Autodesk Fusion 360 part; units mm, degrees
sketch "Sketch1" plane through (0, 0, 0) normal (0, 1, 0) x (1, 0, 0)
  line L0 (-18.22, -14.04) -> (0, -14.04)
  line L1 (0, -14.04) -> (0, 14.04)
  line L2 (0, 14.04) -> (-18.22, 14.04)
  line L3 (-18.22, 14.04) -> (-18.22, -14.04)
  line L4 (0, -5.075) -> (-4, -5.075)
  line L5 (-4, -5.075) -> (-4, -7.75)
  line L6 (-4, -7.75) -> (-14.22, -7.75)
  line L7 (0, 5.075) -> (-4, 5.075)
  line L8 (-4, 5.075) -> (-4, 7.75)
  line L9 (-4, 7.75) -> (-14.22, 7.75)
  line L10 (-14.22, 7.75) -> (-14.22, -7.75)
  line L11 (-18.22, 0) -> (0, 0) construction
  line L12 (-4, -5.075) -> (-4, 5.075) construction
  point P0 (-14.22, 0)
  point P1 (-4, 0)
  dimension "d1" = 28.08
  dimension "d2" = 10.15
  dimension "d3" = 4
  dimension "d4" = 10.22
  dimension "d5" = 15.5
  dimension "d6" = 2.675
  dimension "d7" = 14.22
  dimension "d10" = 4
extrude "Extrude1" add sketch "Sketch1" along normal blind 100 contours L0 L1 L2 L3 L4 L5 L6 L7 L8 L9 L10 makes body 1
sketch "Sketch2" plane through (0, 0, 0) normal (0, 1, 0) x (1, 0, 0)
  line L0 (-4, -7.75) -> (-14.22, -7.75)
  line L1 (-14.22, 7.75) -> (-14.22, -7.75)
  line L2 (-4, 7.75) -> (-14.22, 7.75)
  line L3 (-4, 5.075) -> (-4, 7.75)
  line L4 (0, 5.075) -> (-4, 5.075)
  line L5 (0, -5.075) -> (-4, -5.075)
  line L6 (-4, -5.075) -> (-4, -7.75)
  line L7 (0, -14.04) -> (0, 14.04)
  line L8 (0, 5.075) -> (0, -5.075)
  line L9 (-0.4, -4.675) -> (-4.4, -4.675)
  line L10 (-4.4, -4.675) -> (-4.4, -7.35)
  line L11 (-4.4, -7.35) -> (-13.82, -7.35)
  line L12 (-13.82, 7.35) -> (-13.82, -7.35)
  line L13 (-4.4, 7.35) -> (-13.82, 7.35)
  line L14 (-4.4, 4.675) -> (-4.4, 7.35)
  line L15 (-0.4, 4.675) -> (-4.4, 4.675)
  line L16 (-0.4, 4.675) -> (-0.4, -4.675)
  dimension "d11" = 0.4
extrude "Extrude2" add sketch "Sketch2" along normal mid plane 20 separate body contours L9 L10 L11 L12 L13 L14 L15 L16 makes body 2
sketch "Sketch4" plane through (-13.82, 0, 0) normal (-1, 0, 0) x (0, -1, 0)
  line L0 (10, 7.35) -> (-10, 7.35)
  line L1 (-10, 7.35) -> (-10, -7.35)
  line L2 (-10, -7.35) -> (10, -7.35)
  line L3 (10, -7.35) -> (10, 7.35)
  line L4 (3.3811, 5.8563) -> (-3.3811, 5.8562)
  line L5 (-3.3811, 5.8562) -> (-6.7622, 0)
  line L6 (-6.7622, 0) -> (-3.3811, -5.8563)
  line L7 (-3.3811, -5.8563) -> (3.3811, -5.8563)
  line L8 (3.3811, -5.8563) -> (6.7622, 0)
  line L9 (6.7622, 0) -> (3.3811, 5.8563)
  line L10 (0, 0) -> (10, 0) construction
  circle A0 centre (0, 0) radius 3.378
  dimension "d14" = 11.7125
  dimension "d23" = 6.756
extrude "Extrude3" cut sketch "Sketch4" against normal blind 6.5563 contours L4 L5 L6 L7 L8 L9 bodies 2
extrude "Extrude4" cut sketch "Sketch4" against normal blind 25.66 contours A0 bodies 2
chamfer "Chamfer1" distance 0.4 angle 45 23 edges at (-9.11, 10, 7.35) (-4.4, 0, 7.35) (-9.11, -10, 7.35) (-4.4, 10, 6.0125) (-2.4, 10, 4.675) (-0.4, 10, 0) (-2.4, 10, -4.675) (-4.4, 10, -6.0125) (-9.11, 10, -7.35) (-4.4, 0, -7.35) (-4.4, -10, 6.0125) (-2.4, -10, 4.675) (-0.4, -10, 0) (-2.4, -10, -4.675) (-4.4, -10, -6.0125) (-9.11, -10, -7.35) (-0.4, 0, 4.675) (-0.4, 0, -4.675) (-0.4, 3.1494, -1.2215) (-13.82, 0, 7.35) (-13.82, -10, 0) (-13.82, 0, -7.35) (-13.82, 10, 0) on bodies 2
chamfer "Chamfer2" distance 0.4 angle 45 6 edges at (-13.82, 5.0717, 2.9281) (-13.82, 0, 5.8563) (-13.82, -5.0717, 2.9281) (-13.82, -5.0717, -2.9281) (-13.82, 0, -5.8563) (-13.82, 5.0717, -2.9281) on bodies 2
sketch "Sketch5" plane through (-7.2638, 0, 0) normal (-1, 0, 0) x (0, -1, 0)
  circle A0 centre (0, 0) radius 3.378
  line L0 (6.7622, 0) -> (3.3811, 5.8563)
  line L1 (3.3811, 5.8563) -> (-3.3811, 5.8562)
  line L2 (-3.3811, 5.8562) -> (-6.7622, 0)
  line L3 (-6.7622, 0) -> (-3.3811, -5.8563)
  line L4 (-3.3811, -5.8563) -> (3.3811, -5.8563)
  line L5 (3.3811, -5.8563) -> (6.7622, 0)
extrude "Extrude5" add sketch "Sketch5" against normal blind 0.2 contours A0 bodies 2
hidden bodies 1
equation "d14 = 7 in / 16 + 0.6 mm"
equation "d15 = -7 in / 32 - 1 mm"
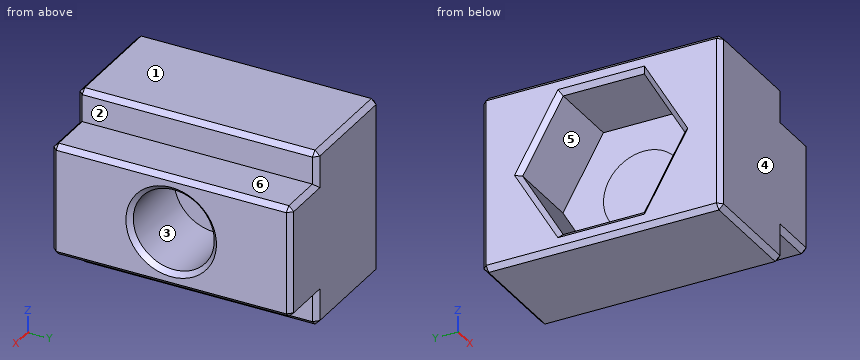
The listing builds one solid part. Answer for the finished solid, in the listing's coordinates (mm). Face numbers are marked on the shaded views. A direction names the side the tool comes from. Give positions to 0.01 mm unless a question says otherwise; leave off trailing zeros. Order: outer loops, then holes, each group sorted by start corner. A loop starts at its lowest first (then second) coordinate and runs counter-clockwise, first axis right, second up. Notation, with made-up numbers: (55, 78.5) - (97, 78.5) arc R24 cw to (97, 91.5) - close; hole circle Ø5 at (71, 50). An arc over 180 degrees is marked (long way). One line per item, written item: value. Start each with the question number.
1) Find the intervals of material crossed by L1, parallel to Z at x = -3.25, y = 0 (3 decimals); L2, parallel to Z at x = -8.25, y = 1; L3, parallel to X at y = -3, z = 3, in increasing order.
2) A cutting plane is placed at C-C on z = 5. Give the vertices of the cut face in (x, y).
3) A tool of negligible diameter and unlimited length cuts with its end or side. For the marked faces 1, 2 and 3, from which of +Z, -Z, +X, -X, +Y, -Y can it reach the whole face along a straight path? Write none if from no direction.
4) A cutting plane is placed at D-D on x = -6.5. Give the vertices of the cut face in (y, z), then the cut area to 3 significant figures.
5) Given pin 1 Ø1.8 at (x, y) = (-2, -2.5) entering from -Z (3 decimals); pin 2 Ø3.5 at (y, z) = (1, -1) entering from -X; pin 3 Ø0.7 at (y, z) = (1.5, -5.5) entering from +X, each flat-ended and moving along its own axis, determine where each tip first touches the part or whether it passes through.
6) A cutting plane is placed at A-A on x = -3. Give the vertices of the cut face in (y, z) (3 decimals).
7) The mould has two halves that part along Y. Classify the marked faces 4, 5 and 6: released by +Y, released by -Y, zero draft, split by the parting line, or undercut.
8) A cutting plane is placed at B-B on y = 0. Give the vertices of the cut face in (x, z) (3 decimals).
Answer sheet:
1. L1: z = -4.675 to -3.378, 3.378 to 4.675
1. L2: z = -7.35 to -5.86, 5.86 to 7.35
1. L3: x = -7.26 to -0.4
2. outline: (-13.82, -9.6) - (-13.42, -10) - (-4.8, -10) - (-4.4, -9.6) - (-4.4, 9.6) - (-4.8, 10) - (-13.42, 10) - (-13.82, 9.6) - (-13.82, 4.34) - (-13.42, 3.88) - (-7.26, 3.88) - (-7.26, -3.88) - (-13.42, -3.88) - (-13.82, -4.34) - close
3. face 1: +Z, +X, -X, +Y, -Y
3. face 2: +Z, +X, +Y, -Y
3. face 3: +X
4. outline: (-10, -6.95) - (-9.6, -7.35) - (9.6, -7.35) - (10, -6.95) - (10, 6.95) - (9.6, 7.35) - (-9.6, 7.35) - (-10, 6.95) - close; hole circle Ø6.76 at (0, 0)
4. area: 258 mm2
5. pin 1: stops at z = -4.675
5. pin 2: stops at x = -7.26
5. pin 3: stops at x = -4.4
6. outline: (-10, -4.275) - (-9.6, -4.675) - (9.6, -4.675) - (10, -4.275) - (10, 4.275) - (9.6, 4.675) - (-9.6, 4.675) - (-10, 4.275) - close; hole circle Ø6.756 at (0, 0)
7. face 4: released by -Y
7. face 5: undercut
7. face 6: zero draft
8. outline: (-13.82, -6.95) - (-13.42, -7.35) - (-4.8, -7.35) - (-4.4, -6.95) - (-4.4, -4.675) - (-0.8, -4.675) - (-0.4, -4.275) - (-0.4, -3.778) - (-0.8, -3.378) - (-7.064, -3.378) - (-7.064, 3.378) - (-0.8, 3.378) - (-0.4, 3.778) - (-0.4, 4.275) - (-0.8, 4.675) - (-4.4, 4.675) - (-4.4, 6.95) - (-4.8, 7.35) - (-13.42, 7.35) - (-13.82, 6.95) - (-13.82, 6.256) - (-13.42, 5.856) - (-7.264, 5.856) - (-7.264, 3.378) - (-7.264, -5.856) - (-13.42, -5.856) - (-13.82, -6.256) - close
